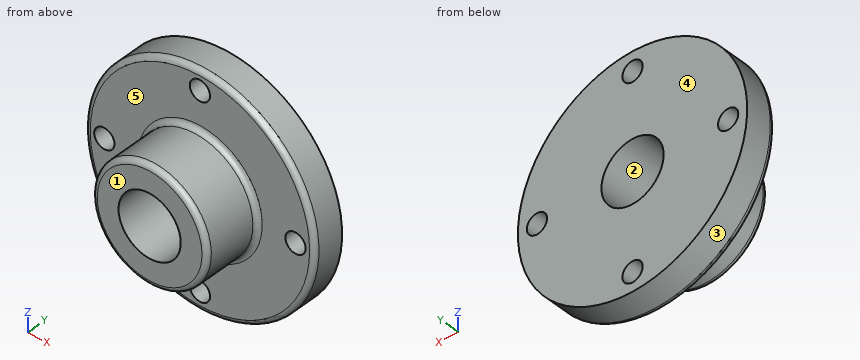
from build123d import *

# Parameters (mm, degrees)
F2_R            = 6.2084574244
F3_DEPTH        = 53.848
F3_COPIES_COUNT = 4
F6_W            = 53.848
F6_H            = 19.0246
F8_R            = 3.048


# Not quite as in the source:
# - a pattern or mirror of a feature is missing from the dataset's text; its kind, count and spacing are read off the source's solid


with BuildPart() as f1:
    # F0 (on Right) → F1 (revolve)
    with BuildSketch(Plane.YZ):
        with BuildLine():
            Line((-19.05, 0), (0, 0))
            Line((0, 0), (0, 70.104))
            Line((0, 70.104), (-16.002, 70.104))
            ThreePointArc((-16.002, 70.104), (-18.1572614691, 69.2112614691), (-19.05, 67.056))
            Line((-19.05, 67.056), (-19.05, 0))
        make_face()
    revolve(axis=Axis((0, -9.525, 0), (0, -1, 0)))

    # F2 (on Front) → F3 (cut)
    with BuildSketch(Plane.XZ):
        with Locations((0, 58.4511086345)):
            Circle(F2_R)
    f3 = extrude(amount=F3_DEPTH, mode=Mode.SUBTRACT)

    # F3_copies: F3 ×4 about axis
    f3_copies_axis = Axis((0, 0, 0), (0, 1, 0))
    for i in range(1, F3_COPIES_COUNT):
        add(f3.rotate(f3_copies_axis, i * 360 / F3_COPIES_COUNT), mode=Mode.SUBTRACT)

    # F4 (on Right) → F5 (revolve)
    with BuildSketch(Plane.YZ):
        with BuildLine():
            Line((-53.848, 0), (0, 0))
            Line((0, 0), (0, 35.052))
            Line((0, 35.052), (-50.8, 35.052))
            ThreePointArc((-50.8, 35.052), (-52.9552614691, 34.1592614691), (-53.848, 32.004))
            Line((-53.848, 32.004), (-53.848, 0))
        make_face()
    revolve(axis=Axis((0, -26.924, 0), (0, -1, 0)))

    # F6 (on Right) → F7 (revolve, cut)
    with BuildSketch(Plane.YZ):
        with Locations((-26.924, 9.5123)):
            Rectangle(F6_W, F6_H)
    revolve(axis=Axis((0, -26.924, 0), (0, -1, 0)), mode=Mode.SUBTRACT)

    # F8
    f8_edges = [f1.edges().sort_by_distance(p)[0] for p in [
        (0, -19.05, -35.052),
    ]]
    fillet(f8_edges, radius=F8_R)


solid = f1.part
For this review, take the finished solid that the model builds, in its own axes (mm). Face numbers are marked on the shaded views. A direction names the side the tool comes from. Give positions to 0.01 mm unless a question says otherwise; leave off trailing zeros. Order: outer loops, then holes, each group sorted by start corner. A loop starts at its lowest first (then second) coordinate and runs counter-clockwise, first axis right, second up. Notation, with made-up numbers: M 37.25,70 L 71.25,70 A15 cw 71.25,91 Z; hole C -38,40.5 d9. An arc over 180 degrees is marked long. Answer in a Markdown table with one row per item. Add a question column.
(1) Mouldability with a two-part tool opening along Z and no side actions: class the marked faces 1, 2 and 3 as +Z half, -Z half, draft (parallel to the pull), parting line (faces both ways), or undercut.
(2) For pin 1 (3 mm diameter, centred on y = -10.5, z = 49, fed in from +X); pin 2 (5 mm diameter, centred on x = 30.5, y = -45.5, fed in from -Z); pin 3 (16 mm diameter, centred on x = 0, z = 58.45, fed in from -Y); pin 4 (7.5 mm diameter, centred on x = -58.45, z = 0, fed in from -Y), all flat-tipped, find the tip position at first contact; note any pin that passes through.
(3) Wall thickness on probe 1 along Z at (x, y) = (0, -39.5); probe 2 along Z at (x, y) = (0, -13.5); probe 3 along Z at (x, y) = (-5, -3.5): over which ranges is each line inside the solid? List them lowest first. Write a range as [from, to].
(4) Consider section B-B on z = 0. State the section outline as (x, y) points.
(5) Consider section A-A on x = 0. State the section outline as (y, z) points.
(6) For the marked faces 4 and 5, list the 3-axis set-ups (+Z, -Z, +X, -X, +Y, -Y) from which the entire face can be reached by the end or side of a thin tool; tool diameter is ignored.
(7) Consider section C-C on y = -28.5. State the section outline as (x, z) points, and give its area (3 significant figures).
Evaluation:
| question | item | result |
|---|---|---|
| 1 | face 1 | draft |
| 1 | face 2 | undercut |
| 1 | face 3 | parting line |
| 2 | pin 1 | stops at x = 51.56 |
| 2 | pin 2 | stops at z = -21.09 |
| 2 | pin 3 | stops at y = -19.05 |
| 2 | pin 4 | passes through |
| 3 | probe 1 | z = [-35.05, -19.02], [19.02, 35.05] |
| 3 | probe 2 | z = [-70.1, -64.66], [-52.24, -19.02], [19.02, 52.24], [64.66, 70.1] |
| 3 | probe 3 | z = [-69.93, -62.13], [-54.77, -18.36], [18.36, 54.77], [62.13, 69.93] |
| 4 | outline | M -70.1,-16 A3.05 ccw -67.06,-19.05 L -64.66,-19.05 L -64.66,0 L -70.1,0 Z; M -52.24,-19.05 L -38.1,-19.05 A3.05 cw -35.05,-22.1 L -35.05,-50.8 A3.05 ccw -32,-53.85 L -19.02,-53.85 L -19.02,0 L -52.24,0 Z; M 19.02,-53.85 L 32,-53.85 A3.05 ccw 35.05,-50.8 L 35.05,-22.1 A3.05 cw 38.1,-19.05 L 52.24,-19.05 L 52.24,0 L 19.02,0 Z; M 64.66,-19.05 L 67.06,-19.05 A3.05 ccw 70.1,-16 L 70.1,0 L 64.66,0 Z |
| 5 | outline | M -53.85,-32 A3.05 ccw -50.8,-35.05 L -22.1,-35.05 A3.05 cw -19.05,-38.1 L -19.05,-52.24 L 0,-52.24 L 0,-19.02 L -53.85,-19.02 Z; M -53.85,19.02 L 0,19.02 L 0,52.24 L -19.05,52.24 L -19.05,38.1 A3.05 cw -22.1,35.05 L -50.8,35.05 A3.05 ccw -53.85,32 Z; M -19.05,-67.06 A3.05 ccw -16,-70.1 L 0,-70.1 L 0,-64.66 L -19.05,-64.66 Z; M -19.05,64.66 L 0,64.66 L 0,70.1 L -16,70.1 A3.05 ccw -19.05,67.06 Z |
| 6 | face 4 | +Z, -Z, +X, -X, +Y |
| 6 | face 5 | -Y |
| 7 | outline | C 0,0 d70.1; hole C 0,0 d38.05 |
| 7 | area | 2,720 mm^2 |
